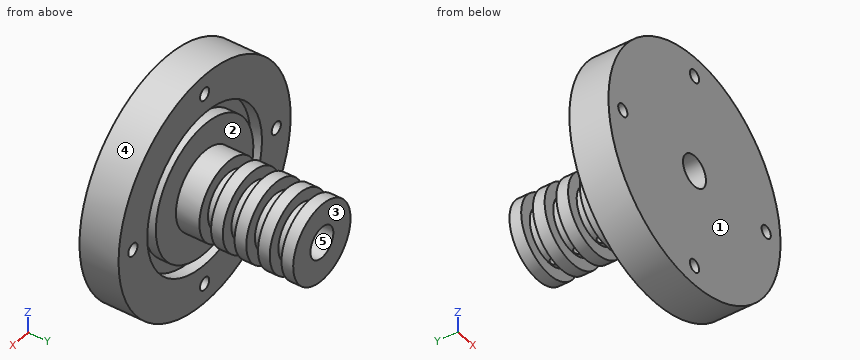
```python
from build123d import *

# Parameters (mm, degrees)
SKETCH5_R          = 1.6
CUT_EXTRUDE2_DEPTH = 10
SKETCH8_R          = 1.25
CUT_EXTRUDE3_DEPTH = 10


with BuildPart() as part:
    # Sketch2 → Revolve1 (revolve)
    with BuildSketch(Plane.XY, mode=Mode.PRIVATE) as revolve1_sk:
        Polygon((4, 35.968329977), (4, -4.031670023), (30, -4.031670023), (30, 5.968329977), (20, 5.968329977), (20, 2.968329977), (17, 2.968329977), (17, 5.968329977), (10, 5.968329977), (10, 11.968329977), (7, 11.968329977), (7, 14.968329977), (10, 14.968329977), (10, 17.968329977), (7, 17.968329977), (7, 20.968329977), (10, 20.968329977), (10, 23.968329977), (7, 23.968329977), (7, 26.968329977), (10, 26.968329977), (10, 29.968329977), (7, 29.968329977), (7, 32.968329977), (10, 32.968329977), (10, 35.968329977), align=None)
    revolve(revolve1_sk.sketch.rotate(Axis((0, 37.555974624, 0), (0, -1, 0)), 90), axis=Axis((0, 37.555974624, 0), (0, -1, 0)))

    # Sketch5 → Cut-Extrude2 (cut)
    with BuildSketch(Plane(origin=(0, 5.968329977, 0), x_dir=(1, 0, 0), z_dir=(0, 1, 0))):
        with Locations(Location((-25, 0, 0), (0, 0, 270))):
            Circle(SKETCH5_R)
        with Locations(Location((0, 25, 0), (0, 0, 270))):
            Circle(SKETCH5_R)
        with Locations(Location((25, 0, 0), (0, 0, 270))):
            Circle(SKETCH5_R)
        with Locations(Location((0, -25, 0), (0, 0, 270))):
            Circle(SKETCH5_R)
    extrude(amount=-CUT_EXTRUDE2_DEPTH, mode=Mode.SUBTRACT)

    # Sketch8 → Cut-Extrude3 (cut)
    with BuildSketch(Plane.XY):
        with Locations((0, 31.468329977)):
            Circle(SKETCH8_R)
        with Locations((0, 25.468329977)):
            Circle(SKETCH8_R)
        with Locations((0, 19.468329977)):
            Circle(SKETCH8_R)
        with Locations((0, 13.468329977)):
            Circle(SKETCH8_R)
    extrude(amount=-CUT_EXTRUDE3_DEPTH, mode=Mode.SUBTRACT)


solid = part.part
```
Here's how the part is built. I have some questions about the finished solid (model axes, mm). Face numbers are marked on the shaded views. A direction names the side the tool comes from. Give positions to 0.01 mm unless a question says otherwise; leave off trailing zeros. Loops run counter-clockwise (first coordinate to the right, second up) from the corner with the lowest first, then second, coordinate; pieces in that order, holes last. Notation, with made-up numbers: (35, 50.5) -> (66, 50.5) arc R32 cw to (66, 79.5) -> close; hole circle Ø3 at (75, 4). An arc over 180 degrees is marked (long way). Use one line per item in the form item = value. Start each with the question number.
1) For P1, Ø8, axis at y = 24.5, z = 4.5, coming from the -X side; P2, Ø12, axis at x = 0.5, y = 16.5, coming from the -Z side; P3, Ø5, axis at y = 25.5, z = -8.5, coming from the +X side, each with a flat end and sliding along its axis, tell me the tip position at first contact or that it passes through.
2) Imagine slicing it at B-B (x = 25). Please give me the cut outline in (y, z), then the cut area to 3 significant figures.
3) Which directions (+Z, -Z, +X, -X, +Y, -Y) give clear straight access to the entire face, cutting with the end or side of a thin tool? Please do the marked faces 1 and 2.
4) Imagine slicing it at C-C (y = 16). Please give me the cut outline in (x, z), then the cut area to 3 significant figures.
5) Imagine slicing it at A-A (z = 0). Count the separate pieces of the cut face and the enclosed holes in it, then the cut area to 3 significant figures.
6) Thinking about a two-plate mould opening in Z: for the marked faces 3, 4 and 5, which applies, +Z half, -Z half, draft (parallel to the pull), parting line (faces both ways), or undercut?
7) Imagine slicing it at D-D (z = 25). Please give me the cut outline in (x, y).
8) Please list where these lines run through material, in increasing order: line 1 along Y through (x, z) = (0, -5); line 2 along Y through (x, z) = (9, -1); line 3 along X through (y, z) = (14, 0).
Check values:
q1.P1 = -9.99
q1.P2 = -10
q1.P3 = 7.62
q2.outline = (-4.03, -16.58) -> (5.97, -16.58) -> (5.97, -1.6) -> (-4.03, -1.6) -> close; (-4.03, 1.6) -> (5.97, 1.6) -> (5.97, 16.58) -> (-4.03, 16.58) -> close
q2.area = 300 mm^2
q3.face_1 = +Z, -Z, +X, -X, -Y
q3.face_2 = +Y
q4.outline = circle Ø20 at (0, 0); hole circle Ø8 at (0, 0)
q4.area = 264 mm^2
q5.separate_pieces = 4
q5.enclosed_holes = 0
q5.area = 726 mm^2
q6.face_3 = draft
q6.face_4 = parting line
q6.face_5 = undercut
q7.outline = (-16.58, -4.03) -> (-1.6, -4.03) -> (-1.6, 5.97) -> (-16.58, 5.97) -> close; (1.6, -4.03) -> (16.58, -4.03) -> (16.58, 5.97) -> (1.6, 5.97) -> close
q8.line_1 = -4.03 to 12.22, 14.72 to 18.22, 20.72 to 24.22, 26.72 to 30.22, 32.72 to 35.97
q8.line_2 = -4.03 to 11.97, 14.97 to 17.97, 20.97 to 23.97, 26.97 to 29.97, 32.97 to 35.97
q8.line_3 = -7 to -4, 4 to 7
